Geometry: see drawing. Coordinates: mm, zero at the bounding-box minimum. A direction names the side the tool comes from. Round coordinates to 2 decimals unless told otherwise and drop trailing zeros. Write each loop counter-clockwise with the first axis right and the second up, starting at its lowest first coordinate (ties: lowest second). Pieces come first, ordered by that corner, then holes. Notation, with made-up numbers: (71, 23) - (92, 23) arc R35 ccw to (92, 56) - close; hole circle Ø3 at (38.5, 51). An arc over 180 degrees is marked (long way). Use a Markdown table: item, result. Add a question column.
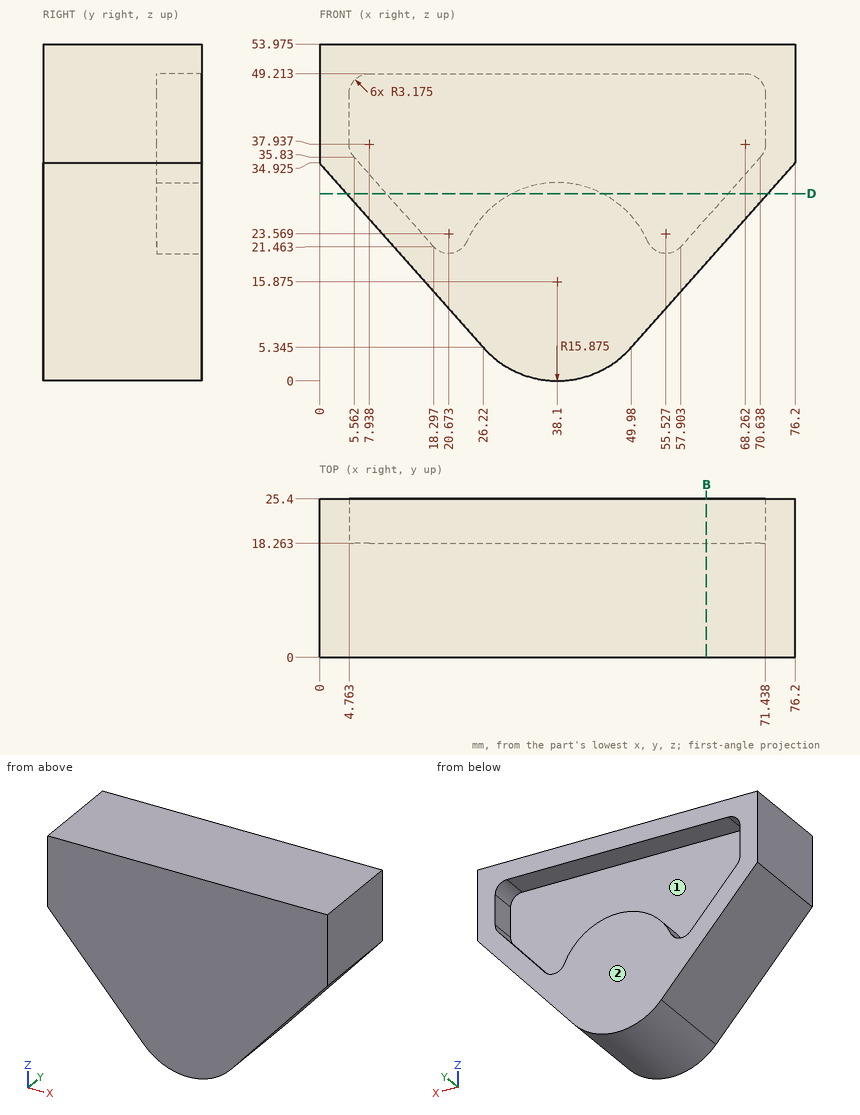
1) Material intervals for L1, parallel to X at y = 18.5, z = 39; L2, parallel to Y at x = 8.5, z = 48; L3, parallel to Z at x = 65, y = 20.25 (1 decimal), sorted ascending. Write a range as from..to.
2) Pin query (flat end, axial travel): P1, Ø2, axis at y = 18, z = 24, coming from the -X side; P2, Ø2, axis at x = 42.5, y = 23, coming from the -Z side; P3, Ø1, axis at x = 64, y = 21.5, coming from the -Z side. Return the tip coordinate at first contact, or that it passes through.
3) Set-up query: the marked faces 1 and 2. Return all of +Z, -Z, +X, -X, +Y, -Y with unobstructed straight access to the full face (end or side cutting, diameter ignored); none if empty.
4) Section B-B, the plane x = 62. Return the cut outline in (y, z) (1 decimal).
5) Section D-D, the plane z = 30. Return the cut outline in (x, y) (1 decimal), then the cut area to 3 significant figures.
Output values:
| question | item | result |
|---|---|---|
| 1 | L1 | x = 0..4.76, 71.44..76.2 |
| 1 | L2 | y = 0..18.26 |
| 1 | L3 | z = 22.3..29.5, 49.2..54 |
| 2 | P1 | stops at x = 8.8 |
| 2 | P2 | stops at z = 0.37 |
| 2 | P3 | stops at z = 20.6 |
| 3 | face 1 | +Y |
| 3 | face 2 | +Z, -Z, +X, -X, +Y |
| 4 | outline | (0, 18.9) - (25.4, 18.9) - (25.4, 26.1) - (18.3, 26.1) - (18.3, 49.2) - (25.4, 49.2) - (25.4, 54) - (0, 54) - close |
| 5 | outline | (4.4, 0) - (71.8, 0) - (71.8, 25.4) - (65.5, 25.4) - (65.5, 18.3) - (45.3, 18.3) - (45.3, 25.4) - (30.9, 25.4) - (30.9, 18.3) - (10.7, 18.3) - (10.7, 25.4) - (4.4, 25.4) - close |
| 5 | area | 1,430 mm^2 |
